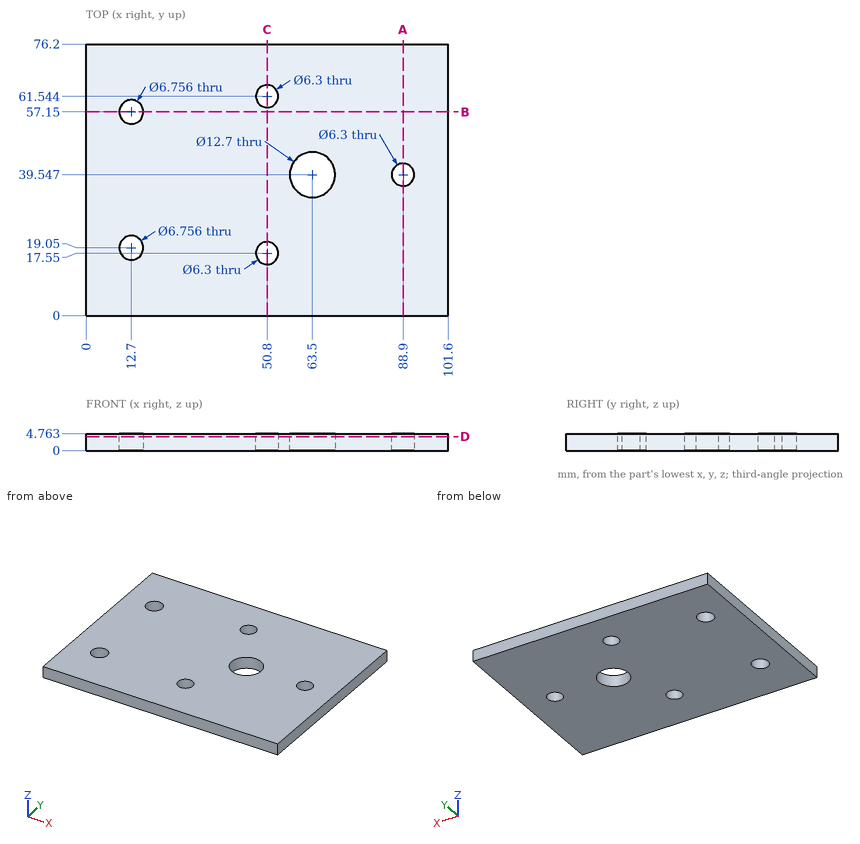
Input: dimensioned drawing with shaded views. Units: mm. Origin: part minimum x, y, z. Round coordinates to 2 decimals unless told otherwise and drop trailing zeros. Order: outer loops, then holes, each group sorted by start corner. A loop starts at its lowest first (then second) coordinate and runs counter-clockwise, first axis right, second up.
1. Cut plane C-C, the plane x = 50.8. Output: boundary loops of the cut face in (y, z).
The answers:
outline: (0, 0) - (14.4, 0) - (14.4, 4.76) - (0, 4.76) - close; (20.7, 0) - (58.39, 0) - (58.39, 4.76) - (20.7, 4.76) - close; (64.69, 0) - (76.2, 0) - (76.2, 4.76) - (64.69, 4.76) - close
2. Pin query (flat end, axial travel): P1, Ø16.5, axis at x = 63.5, y = 39.55, coming from the +Z side. Return the tip coordinate at first contact, or that it passes through.
The answers:
P1: stops at z = 4.76
3. Cut plane D-D, the plane z = 3.95. Output: boundary loops of the cut face in (x, y), then the cut area to 3 significant figures.
The answers:
outline: (0, 0) - (101.6, 0) - (101.6, 76.2) - (0, 76.2) - close; hole circle Ø6.76 at (12.7, 19.05); hole circle Ø6.76 at (12.7, 57.15); hole circle Ø6.3 at (50.8, 17.55); hole circle Ø6.3 at (50.8, 61.54); hole circle Ø12.7 at (63.5, 39.55); hole circle Ø6.3 at (88.9, 39.55)
area: 7,450 mm2
4. Cut plane B-B, the plane y = 57.15. Output: boundary loops of the cut face in (x, z).
The answers:
outline: (0, 0) - (9.32, 0) - (9.32, 4.76) - (0, 4.76) - close; (16.08, 0) - (101.6, 0) - (101.6, 4.76) - (16.08, 4.76) - close
5. Material intervals for line 1 (Y direction, x = 50.8, z = 3.15); line 2 (Y direction, x = 12.7, z = 2.6); line 3 (Y direction, x = 89, z = 2.9) (1 decimal), sorted ascending.
The answers:
line 1: y = 0 to 14.4, 20.7 to 58.39, 64.69 to 76.2
line 2: y = 0 to 15.67, 22.43 to 53.77, 60.53 to 76.2
line 3: y = 0 to 36.4, 42.7 to 76.2
6. Cut plane A-A, the plane x = 88.9. Output: boundary loops of the cut face in (y, z).
The answers:
outline: (0, 0) - (36.4, 0) - (36.4, 4.76) - (0, 4.76) - close; (42.7, 0) - (76.2, 0) - (76.2, 4.76) - (42.7, 4.76) - close
